The listing builds one solid part. Answer for the finished solid, in the listing's coordinates (mm). Face numbers are marked on the shaded views. A direction names the side the tool comes from. Coordinates: 2 decimals unless noted, no trailing zeros. Order: outer loops, then holes, each group sorted by start corner. A loop starts at its lowest first (then second) coordinate and runs counter-clockwise, first axis right, second up. Notation, with made-up numbers: M 41.25,17.5 L 64.25,17.5 A28 cw 64.25,44.5 Z; hole C -35.75,18 d4. An arc over 180 degrees is marked long. One line per item, written item: value. Start each with the question number.
Q1. The part is cut by section B-B on z = -92. Give the vertices of the cut face in (x, y), then the cut area to 3 significant figures.
Q2. For the marked faces 4 and 5, determine the directions among +Z, -Z, +X, -X, +Y, -Y from which every point of the face is accessible in a straight line to the end or side of a thin tool.
Q3. Straight lines are drawn through the part: line 1 along X through (y, z) = (125, 73); line 2 along Y through (x, z) = (-361.5, -92.5). For each, find the intervals that lie inside material, in ascending order. Write a range as [from, to].
Q4. Determine the mould class of the marked faces 1, 2 and 3 for opening direction X: pulls with the +X half, pulls with the -X half, needs draft (parallel to the pull), parting line crosses it, or undercut.
Q5. The part is cut by section A-A on y = 80.5. Give the vertices of the cut face in (x, z).
Q6. Each of these flat-tipped pins is pushed along its axis until it touches: pin 1 Ø10.5 at (x, z) = (228, -130) entering from +Y; pin 2 Ø5 at (y, z) = (198, 10) entering from -X; pin 3 Ø3 at (x, z) = (47.72, 130.35) entering from -Y; pin 4 Ø8.5 at (x, z) = (227.64, -131.82) entering from +Y. Where does it stop, or does it pass through?
Q7. The part is cut by section C-C on x = -28. Give the vertices of the cut face in (y, z), then the cut area to 3 significant figures.
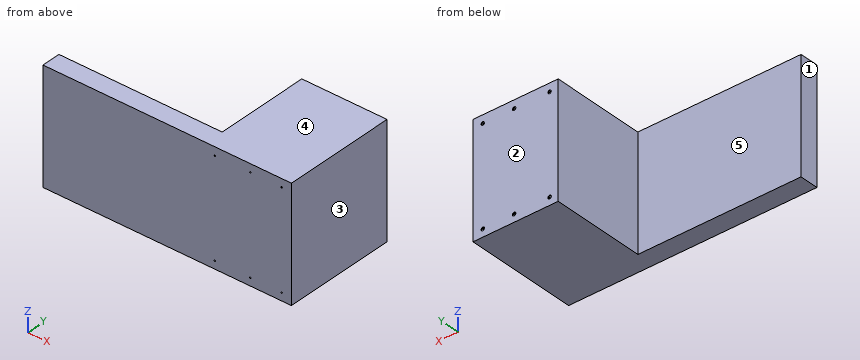
```python
from build123d import *

# Parameters (mm, degrees)
SKETCH1_W                                   = 508
SKETCH1_H                                   = 304.8
BOSS_EXTRUDE1_DEPTH                         = 50.8
SKETCH2_W                                   = 229.423241107
SKETCH2_H                                   = 304.8
BOSS_EXTRUDE2_DEPTH                         = 254
BOSS_EXTRUDE3_DEPTH                         = 304.8
CBORE_FOR_M3_HEX_HEAD_CAP_SCREW1_AT_2_COUNT = 2
CBORE_FOR_M3_HEX_HEAD_CAP_SCREW1_AT_2_PITCH = 95.46630017
CBORE_FOR_M3_HEX_HEAD_CAP_SCREW1_AT_3_COUNT = 2
CBORE_FOR_M3_HEX_HEAD_CAP_SCREW1_AT_3_PITCH = 179.917258012
CBORE_FOR_M3_HEX_HEAD_CAP_SCREW1_AT_4_COUNT = 2
CBORE_FOR_M3_HEX_HEAD_CAP_SCREW1_AT_4_PITCH = 317.963495132
CBORE_FOR_M3_HEX_HEAD_CAP_SCREW1_AT_5_COUNT = 2
CBORE_FOR_M3_HEX_HEAD_CAP_SCREW1_AT_5_PITCH = 279.006055443
CBORE_FOR_M3_HEX_HEAD_CAP_SCREW1_AT_6_COUNT = 2
CBORE_FOR_M3_HEX_HEAD_CAP_SCREW1_AT_6_PITCH = 262.165147389


with BuildPart() as part:
    # Sketch1 → Boss-Extrude1 (new body)
    with BuildSketch(Plane(origin=(0, 0, 0), x_dir=(1, 0, 0), z_dir=(0, 1, 0))):
        Rectangle(SKETCH1_W, SKETCH1_H)
    extrude(amount=BOSS_EXTRUDE1_DEPTH)

    # Sketch2 → Boss-Extrude2 (add)
    with BuildSketch(Plane(origin=(0, 50.8, 0), x_dir=(1, 0, 0), z_dir=(0, 1, 0))):
        with Locations((139.288379447, 0)):
            Rectangle(SKETCH2_W, SKETCH2_H)
    extrude(amount=BOSS_EXTRUDE2_DEPTH)

    # Sketch3 → Boss-Extrude3 (add)
    with BuildSketch(Plane.XY.offset(152.4)):
        Polygon((-254, 0), (-414.851586113, 0), (-414.851586113, 50.8), (-254, 50.8), (24.576758893, 50.8), (24.576758893, 304.8), (254, 304.8), (254, 0), align=None)
    extrude(amount=-BOSS_EXTRUDE3_DEPTH)

    # Sketch6 → CBORE for M3 Hex Head Cap Screw1 (revolve, cut)
    with BuildSketch(Plane(origin=(47.719356018, 304.8, -131.81692985), x_dir=(0, 0, 1), z_dir=(1, 0, 0))):
        Polygon((0, 0), (0, 304.8), (1.8, 304.8), (1.8, 2), (4.6755, 2), (4.6755, 0.025), (4.7005, 0), align=None)
    cbore_for_m3_hex_head_cap_screw1 = revolve(axis=Axis((47.719356018, 311.15, -131.81692985), (0, -1, 0)), mode=Mode.SUBTRACT)

    # CBORE for M3 Hex Head Cap Screw1 at 2: CBORE for M3 Hex Head Cap Screw1 ×2
    with Locations(*[(i * CBORE_FOR_M3_HEX_HEAD_CAP_SCREW1_AT_2_PITCH, 0, 0) for i in range(1, CBORE_FOR_M3_HEX_HEAD_CAP_SCREW1_AT_2_COUNT)]):
        add(cbore_for_m3_hex_head_cap_screw1, mode=Mode.SUBTRACT)

    # CBORE for M3 Hex Head Cap Screw1 at 3: CBORE for M3 Hex Head Cap Screw1 ×2
    with Locations(*[(i * CBORE_FOR_M3_HEX_HEAD_CAP_SCREW1_AT_3_PITCH, 0, 0) for i in range(1, CBORE_FOR_M3_HEX_HEAD_CAP_SCREW1_AT_3_COUNT)]):
        add(cbore_for_m3_hex_head_cap_screw1, mode=Mode.SUBTRACT)

    # CBORE for M3 Hex Head Cap Screw1 at 4: CBORE for M3 Hex Head Cap Screw1 ×2
    with Locations(*[Vector(0.565842497, 0, 0.824513353) * (i * CBORE_FOR_M3_HEX_HEAD_CAP_SCREW1_AT_4_PITCH) for i in range(1, CBORE_FOR_M3_HEX_HEAD_CAP_SCREW1_AT_4_COUNT)]):
        add(cbore_for_m3_hex_head_cap_screw1, mode=Mode.SUBTRACT)

    # CBORE for M3 Hex Head Cap Screw1 at 5: CBORE for M3 Hex Head Cap Screw1 ×2
    with Locations(*[Vector(0.342165692, 0, 0.939639632) * (i * CBORE_FOR_M3_HEX_HEAD_CAP_SCREW1_AT_5_PITCH) for i in range(1, CBORE_FOR_M3_HEX_HEAD_CAP_SCREW1_AT_5_COUNT)]):
        add(cbore_for_m3_hex_head_cap_screw1, mode=Mode.SUBTRACT)

    # CBORE for M3 Hex Head Cap Screw1 at 6: CBORE for M3 Hex Head Cap Screw1 ×2
    with Locations(*[(0, 0, i * CBORE_FOR_M3_HEX_HEAD_CAP_SCREW1_AT_6_PITCH) for i in range(1, CBORE_FOR_M3_HEX_HEAD_CAP_SCREW1_AT_6_COUNT)]):
        add(cbore_for_m3_hex_head_cap_screw1, mode=Mode.SUBTRACT)


solid = part.part
```
Output:
1. outline: M -414.85,0 L 254,0 L 254,304.8 L 24.58,304.8 L 24.58,50.8 L -414.85,50.8 Z
1. area: 92,300 mm^2
2. face 4: +Z, +X, -X, +Y, -Y
2. face 5: +Z, -Z, -X, +Y
3. line 1: x = [24.58, 254]
3. line 2: y = [0, 50.8]
4. face 1: pulls with the -X half
4. face 2: needs draft
4. face 3: pulls with the +X half
5. outline: M 24.58,-152.4 L 254,-152.4 L 254,152.4 L 24.58,152.4 Z; hole C 47.72,-131.82 d3.6; hole C 47.72,130.35 d3.6; hole C 143.19,-131.82 d3.6; hole C 143.19,130.35 d3.6; hole C 227.64,-131.82 d3.6; hole C 227.64,130.35 d3.6
6. pin 1: stops at y = 304.8
6. pin 2: stops at x = 24.58
6. pin 3: passes through
6. pin 4: stops at y = 302.8
7. outline: M 0,-152.4 L 50.8,-152.4 L 50.8,152.4 L 0,152.4 Z
7. area: 15,500 mm^2
